Here's how the part is built. I have some questions about the finished solid (model axes, mm). Coordinates: 2 decimals unless noted, no trailing zeros. Write each loop counter-clockwise with the first axis right and the second up, starting at its lowest first coordinate (ties: lowest second). Pieces come first, ordered by that corner, then holes.
(1) Please list where these lines run through material, in increasing order: probe 1 along X at (y, z) = (12.5, 0.05); probe 2 along Z at (x, y) = (0.8, 7.5); probe 3 along Z at (x, y) = (0.65, 14).
(2) Imagine slicing it at A-A, the plane z = 0. List the corners of the cut face in (x, y) for me, plus the area to 3 significant figures.
(3) For pin 1 Ø1.5 at (x, y) = (-1.5, 10.5) entering from -Z; pin 2 Ø1 at (x, z) = (-0.5, -1) entering from -Y, each with a flat end and sliding along its axis, tell me the tip position at first contact or that it passes through.
(4) Thinking about a two-plate mould opening in X: for faces 1 (the cylindrical face through (0.45, 7.5, 1.43)), 2 (the flat face through (-0.99, 7.5, -1.74)), 3 (the flat face through (0, 15, 2)), 4 (the flat face through (0.99, 7.5, 1.74)), which applies, released by +X, released by -X, zero draft, split by the parting line, or undercut?
(5) Imagine slicing it at B-B, the plane y = 5. List the corners of the cut face in (x, z) for me.
```python
from build123d import *

# Parameters (mm, degrees)
ESQUISSE1_R        = 1.5
BOSS_EXTRU_1_DEPTH = 15
CHANFREIN1_SIZE    = 0.2


with BuildPart() as part:
    # Esquisse1 → Boss.-Extru.1 (new body)
    with BuildSketch(Plane(origin=(0, 0, 0), x_dir=(1, 0, 0), z_dir=(0, 1, 0))):
        Polygon((0, -2.309401077), (2, -1.154700538), (2, 1.154700538), (0, 2.309401077), (-2, 1.154700538), (-2, -1.154700538), align=None)
        with Locations(Location((0, 0, 0), (0, 0, 270))):
            Circle(ESQUISSE1_R, mode=Mode.SUBTRACT)
    extrude(amount=BOSS_EXTRU_1_DEPTH)

    # Chanfrein1
    chanfrein1_edges = [part.edges().sort_by_distance(p)[0] for p in [
        (0, 0, -1.5),
        (-2, 0, 0),
        (-1, 0, -1.732050808),
        (1, 0, -1.732050808),
        (2, 0, 0),
        (1, 0, 1.732050808),
        (-1, 0, 1.732050808),
    ]]
    chamfer(chanfrein1_edges, length=CHANFREIN1_SIZE)


solid = part.part
```
Recorded:
1. probe 1: x = -2 to -1.5, 1.5 to 2
1. probe 2: z = -1.85 to -1.27, 1.27 to 1.85
1. probe 3: z = -1.93 to -1.35, 1.35 to 1.93
2. outline: (-2, 0.2) - (-1.8, 0) - (-1.7, 0) - (-1.5, 0.2) - (-1.5, 15) - (-2, 15) - close; (1.5, 0.2) - (1.7, 0) - (1.8, 0) - (2, 0.2) - (2, 15) - (1.5, 15) - close
2. area: 14.9 mm2
3. pin 1: stops at z = -1.88
3. pin 2: stops at y = 0.08
4. face 1: undercut
4. face 2: released by -X
4. face 3: zero draft
4. face 4: released by +X
5. outline: (-2, -1.15) - (0, -2.31) - (2, -1.15) - (2, 1.15) - (0, 2.31) - (-2, 1.15) - close; hole circle Ø3 at (0, 0)
